Check sheet for the modelled part. Datum: model origin and axes. Units: mm. Face numbers are marked on the shaded views. A direction names the side the tool comes from. Give positions to 0.01 mm unless a question says otherwise; leave off trailing zeros. Order: outer loops, then holes, each group sorted by start corner. A loop starts at its lowest first (then second) coordinate and runs counter-clockwise, first axis right, second up. Notation, with made-up numbers: (-2.75, 23) -> (44.25, 23) arc R28 ccw to (44.25, 41) -> close; hole circle Ø1 at (64, 18). An arc over 180 degrees is marked (long way). One line per question, with ' | ' between items.
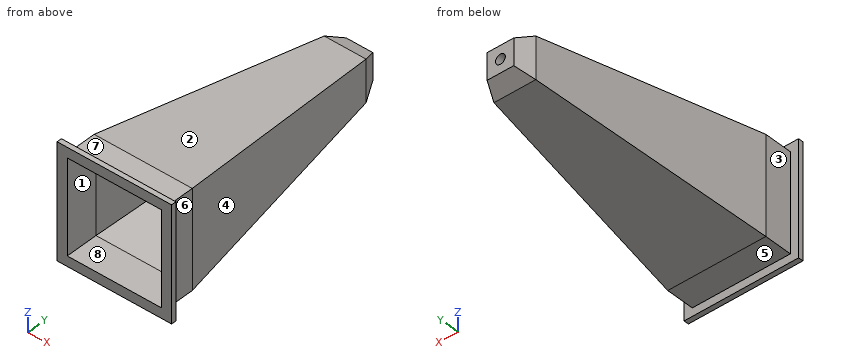
Autodesk Inventor part; units mm, degrees
ref_plane "YZ Plane" through (0, 0, 0) normal (1, 0, 0) x (0, 1, 0)
ref_plane "XZ Plane" through (0, 0, 0) normal (0, 1, 0) x (-1, 0, 0)
ref_plane "XY Plane" through (0, 0, 0) normal (0, 0, 1) x (1, 0, 0)
sketch "Sketch1" plane through (0, 0, 0) normal (0, 1, 0) x (-1, 0, 0)
  line L0 (0, 0) -> (60, 0)
  line L1 (60, 0) -> (60, -60)
  line L2 (60, -60) -> (0, -60)
  line L3 (0, -60) -> (0, 0)
  point P0 (30, -60)
  point P1 (0, -30)
  dimension "d1" = 60
extrude "Extrusion1" add sketch "Sketch1" against normal blind 20
extrude "Extrusion2" add sketch "Sketch1" along normal blind 140 draft -7
shell "Shell1" thickness 1.2 removed faces 1 at (-20, -20, -20)
sketch "Sketch2" plane through (0, 140, 0) normal (0, 1, 0) x (1, 0, 0)
  line L0 (-17.1898, 42.8102) -> (-17.1898, 17.1898)
  line L1 (-42.8102, 42.8102) -> (-17.1898, 42.8102)
  line L2 (-42.8102, 17.1898) -> (-42.8102, 42.8102)
  line L3 (-17.1898, 17.1898) -> (-42.8102, 17.1898)
  circle A0 centre (-30, 30) radius 3
  point P0 (0, 0)
  point P1 (-30, 42.8102)
  point P2 (-42.8102, 30)
  dimension "d7" = 6
extrude "Extrusion4" add sketch "Sketch2" along normal blind 10 draft -25 contours L0 L3 L2 L1 | A0
extrude "Extrusion3" cut sketch "Sketch2" along normal mid plane 25.4 contours A0
sketch "Sketch4" plane through (0, -20, 0) normal (0, -1, 0) x (1, 0, 0)
  line L0 (-65, -65) -> (5, -65)
  line L1 (5, -65) -> (5, 5)
  line L2 (5, 5) -> (-65, 5)
  line L3 (-65, 5) -> (-65, -65)
  line L4 (-58.8, -1.2) -> (-1.2, -1.2)
  line L5 (-1.2, -1.2) -> (-1.2, -58.8)
  line L6 (-58.8, -58.8) -> (-58.8, -1.2)
  line L7 (-1.2, -58.8) -> (-58.8, -58.8)
  point P0 (0, 0)
  point P1 (-30, 5)
  point P2 (-30, -1.2)
  point P3 (5, -30)
  point P4 (-1.2, -30)
  dimension "d16" = 70
extrude "Extrusion6" add sketch "Sketch4" against normal blind 3
properties part number "VRSPAD-144 illumination box"
Q1. Access from +Z, -Z, +X, -X, +Y, -Y to the whole of each face (thin tool, end or side, straight path). Record for the marked faces 1, 2, 3, 4 and 5.
Result sheet:
face 1: -Y | face 2: +Z, +X, -X, +Y | face 3: +Z, -Z, -X, +Y | face 4: +Z, -Z, +X, +Y | face 5: -Z, +X, -X, +Y
Q2. Section check D-D (x = -48). Enter the section's corners in (y, z), and give its area (3 significant figures).
Result sheet:
outline: (-20, -65) -> (-17, -65) -> (-17, -60) -> (0, -60) -> (97.73, -48) -> (97.73, -12) -> (0, 0) -> (-17, 0) -> (-17, 5) -> (-20, 5) -> (-20, -1.2) -> (-0.07, -1.2) -> (87.89, -12) -> (87.89, -48) -> (-0.07, -58.8) -> (-20, -58.8) -> close | area: 657 mm2
Q3. Depth check by flat-ended pin: pin 1 Ø1.5 at (x, z) = (-20.5, -39.5) entering from -Y; pin 2 Ø10 at (y, z) = (-10, -23.5) entering from +X; pin 3 Ø2 at (x, y) = (-36, 56) entering from +Z. Enter the tip coordinate at first touch or a pass-through.
Result sheet:
pin 1: stops at y = 138.8 | pin 2: stops at x = 0 | pin 3: stops at z = -6.75
Q4. Mould release check, pull along Z, two halves, no side actions. Record for the marked faces 6, 7 and 8: pulls with the +Z half, pulls with the -Z half, needs draft (parallel to the pull), parting line crosses it, or undercut.
Result sheet:
face 6: needs draft | face 7: pulls with the +Z half | face 8: undercut
Q5. Thickness scan on line 1 (Z direction, x = -39.5, y = 104.5); line 2 (Z direction, x = -30, y = 144); line 3 (X direction, y = 147.75, z = -30). Record the ranges inside material, lowest first.
Result sheet:
line 1: z = -47.17 to -45.96, -14.04 to -12.83 | line 2: z = -40.94 to -33, -27 to -19.06 | line 3: x = -39.2 to -33, -27 to -20.8
Q6. Section check C-C (y = -7). Enter the section's corners in (x, z), and give its area (3 significant figures).
Result sheet:
outline: (-60, -60) -> (0, -60) -> (0, 0) -> (-60, 0) -> close; hole (-58.8, -58.8) -> (-1.2, -58.8) -> (-1.2, -1.2) -> (-58.8, -1.2) -> close | area: 282 mm2
